Part model, mm, in its own coordinate system. Coordinates: 2 decimals unless noted, no trailing zeros. Loops run counter-clockwise (first coordinate to the right, second up) from the corner with the lowest first, then second, coordinate; pieces in that order, holes last. Notation, with made-up numbers: (22, 60) - (26, 60) arc R16 ccw to (26, 72) - close; hole circle Ø6 at (15.5, 56.25). An arc over 180 degrees is marked (long way). Use a Markdown table: item, result. Add a question column.
1. Drop flat-ended pins along their axis: pin 1 (4 mm diameter, centred on y = -46, z = 50, fed in from +X); pin 2 (8 mm diameter, centred on x = -1.5, z = 50.5, fed in from -Y); pin 3 (6 mm diameter, centred on y = -29, z = 45, fed in from -X). Give the stop position or say it passes through.
2. Band-saw the part on A-A, the plane y = -81.5. Give the cut face in (x, z).
3. Pull direction X, two halves, no side cores. Call faces 1 (the flat face through (12, -101.6, 2)), 2 (the cylindrical face through (-51.171, -51.511, 50.555)), 3 (the cylindrical face through (52.45, -50.09, 49.69)): pulls with the +X half, pulls with the -X half, needs draft (parallel to the pull), parting line crosses it, or undercut.
4. Band-saw the part on C-C, the plane x = -43. Give the cut face in (y, z).
5. Band-saw the part on B-B, the plane z = -31.5. Give the cut face in (x, y), plus the area to 3 significant figures.
6. Wall check: probe 1 along Y at (x, z) = (40.5, -43); probe 2 along X at (y, z) = (-84, 39); probe 3 along X at (y, z) = (-54, 55) (3 decimals). Give the ranges that are in metal, low to high. Write a range as [from, to].
from build123d import *

# Parameters (mm, degrees)
F0_W        = 145.98980546
F0_H        = 145.0418308377
F1_DEPTH    = 101.6
F2_R        = 76.2
F3_T1_DEPTH = 481.2494898574
F5_DEPTH    = 2.54


# Not quite as in the source:
# - a fillet or chamfer that OpenCascade refuses, or shapes differently, is made with other operations: its cross-section is extruded or revolved along the edge and cut away or added


with BuildPart() as f1:
    # F0 (on Front) → F1 (new body)
    with BuildSketch(Plane.XZ):
        with Locations((0.0947937369, 0.9479857981)):
            Rectangle(F0_W, F0_H)
    extrude(amount=F1_DEPTH)

    # F2
    f2_edges = [f1.edges().sort_by_distance(p)[0] for p in [
        (-72.900109, -50.8, 73.468901),
    ]]
    fillet(f2_edges, radius=F2_R)

    # F3: fillet of radius 76.2 on 1 edges, made by hand

    # F3_s2 → F3_t1 (cut)
    with BuildSketch(Plane.XZ.offset(-189.8247449287)):
        with BuildLine():
            ThreePointArc((3.2998910069, 73.468901217), (52.9918213106, 49.1044140169), (73.0896964669, -2.4609967545))
            Line((73.0896964669, -2.4609967545), (73.0896964669, 73.468901217))
            Line((73.0896964669, 73.468901217), (3.2998910069, 73.468901217))
        make_face()
    extrude(amount=F3_T1_DEPTH, mode=Mode.SUBTRACT)

    # F4 (on face) → F5 (join)
    with BuildSketch(Plane.XZ.offset(101.6)):
        with BuildLine():
            add(Edge.make_bspline(
                [(40.2893982828, -52.0444214344), (40.2893982828, -38.976719833), (-20.1446991414, -45.5105706337), (-80.5787965655, -52.0444214344), (-20.1446991414, -58.5782722351), (40.2893982828, -65.1121230358), (40.2893982828, -52.0444214344)],
                knots=[0, 0, 0, 2.0943951024, 2.0943951024, 4.1887902048, 4.1887902048, 6.2831853072, 6.2831853072, 6.2831853072], degree=2, weights=[1, 0.5, 1, 0.5, 1, 0.5, 1]))
        make_face()
    extrude(amount=F5_DEPTH)


solid = f1.part
Geometry check:
| question | item | result |
|---|---|---|
| 1 | pin 1 | stops at x = 53.99 |
| 1 | pin 2 | stops at y = -101.6 |
| 1 | pin 3 | stops at x = -58.39 |
| 2 | outline | (-72.9, -71.57) - (73.09, -71.57) - (73.09, -2.46) arc R76.2 ccw to (3.3, 73.47) arc R76.2 ccw to (-72.9, -2.73) - close |
| 3 | face 1 | needs draft |
| 3 | face 2 | pulls with the -X half |
| 3 | face 3 | pulls with the +X half |
| 4 | outline | (-101.6, -71.57) - (0, -71.57) - (0, 57.79) - (-101.6, 57.79) - close |
| 5 | outline | (-72.9, -101.6) - (73.09, -101.6) - (73.09, 0) - (-72.9, 0) - close |
| 5 | area | 14,800 mm^2 |
| 6 | probe 1 | y = [-101.6, 0] |
| 6 | probe 2 | x = [-60.46, 60.82] |
| 6 | probe 3 | x = [-46.435, 46.936] |
